from build123d import *

# Parameters (mm, degrees)
SKETCH1_W                                    = 20
SKETCH1_H                                    = 40
BOSS_EXTRUDE1_DEPTH                          = 3
CSK_FOR_M3_HEX_SOCKET_COUNTERSUNK_CA_2_COUNT = 2
CSK_FOR_M3_HEX_SOCKET_COUNTERSUNK_CA_2_PITCH = 10
CSK_FOR_M3_HEX_SOCKET_COUNTERSUNK_CA_3_COUNT = 2
CSK_FOR_M3_HEX_SOCKET_COUNTERSUNK_CA_3_PITCH = 18.027756377
CSK_FOR_M3_HEX_SOCKET_COUNTERSUNK_CA_4_COUNT = 2
CSK_FOR_M3_HEX_SOCKET_COUNTERSUNK_CA_4_PITCH = 15
M2_TAPPED_HOLE1_D                            = 1.6
BOSS_EXTRUDE2_DEPTH                          = 3
SKETCH7_W                                    = 30
SKETCH7_H                                    = 80.053183591
SKETCH7_R                                    = 2.65
BOSS_EXTRUDE3_DEPTH                          = 3
SKETCH8_R                                    = 2.65
BOSS_EXTRUDE4_DEPTH                          = 3
SKETCH9_R                                    = 2.6
CUT_EXTRUDE1_DEPTH                           = 4


with BuildPart() as part:
    # Sketch1 → Boss-Extrude1 (new body)
    with BuildSketch(Plane.XY):
        Rectangle(SKETCH1_W, SKETCH1_H)
    extrude(amount=BOSS_EXTRUDE1_DEPTH)

    # Sketch3 → CSK for M3 Hex Socket Countersunk Cap Screw1 (revolve, cut)
    with BuildSketch(Plane(origin=(-5, 0, 3), x_dir=(0, -1, 0), z_dir=(1, 0, 0))):
        Polygon((0, 0), (0, 3), (1.7, 3), (1.7, 1.66), (3.36, 0), align=None)
    csk_for_m3_hex_socket_countersunk_cap_sc = revolve(axis=Axis((-5, 0, 9.35), (0, 0, -1)), mode=Mode.SUBTRACT)

    # CSK for M3 Hex Socket Countersunk Ca 2: CSK for M3 Hex Socket Countersunk Cap Screw1 ×2
    with Locations(*[(i * CSK_FOR_M3_HEX_SOCKET_COUNTERSUNK_CA_2_PITCH, 0, 0) for i in range(1, CSK_FOR_M3_HEX_SOCKET_COUNTERSUNK_CA_2_COUNT)]):
        add(csk_for_m3_hex_socket_countersunk_cap_sc, mode=Mode.SUBTRACT)

    # CSK for M3 Hex Socket Countersunk Ca 3: CSK for M3 Hex Socket Countersunk Cap Screw1 ×2
    with Locations(*[Vector(0.554700196, -0.832050294, 0) * (i * CSK_FOR_M3_HEX_SOCKET_COUNTERSUNK_CA_3_PITCH) for i in range(1, CSK_FOR_M3_HEX_SOCKET_COUNTERSUNK_CA_3_COUNT)]):
        add(csk_for_m3_hex_socket_countersunk_cap_sc, mode=Mode.SUBTRACT)

    # CSK for M3 Hex Socket Countersunk Ca 4: CSK for M3 Hex Socket Countersunk Cap Screw1 ×2
    with Locations(*[(0, -i * CSK_FOR_M3_HEX_SOCKET_COUNTERSUNK_CA_4_PITCH, 0) for i in range(1, CSK_FOR_M3_HEX_SOCKET_COUNTERSUNK_CA_4_COUNT)]):
        add(csk_for_m3_hex_socket_countersunk_cap_sc, mode=Mode.SUBTRACT)

    # M2 Tapped Hole1 (through all)
    with Locations(Plane.XY.offset(3)):
        with Locations((0, 15), (0, 0), (0, -15)):
            Hole(M2_TAPPED_HOLE1_D / 2)

    # Sketch6 → Boss-Extrude2 (add)
    with BuildSketch(Plane.XY.offset(3)):
        Polygon((-10, 4), (-41, 4), (-41, 32), (10, 32), (10, 20), (-10, 20), align=None)
    extrude(amount=-BOSS_EXTRUDE2_DEPTH)

    # Sketch7 → Boss-Extrude3 (add)
    with BuildSketch(Plane.XY.offset(3)):
        with Locations((-10, 72.026591795)):
            Rectangle(SKETCH7_W, SKETCH7_H)
        with Locations((-19, 106.053183591)):
            Circle(SKETCH7_R, mode=Mode.SUBTRACT)
    extrude(amount=-BOSS_EXTRUDE3_DEPTH)

    # Sketch8 → Boss-Extrude4 (add)
    with BuildSketch(Plane.XY.offset(3)):
        Polygon((-25, 4), (-25, -35.5), (10, -35.5), (10, -20), (-10, -20), (-10, 4), align=None)
        with Locations((-19, -29.5)):
            Circle(SKETCH8_R, mode=Mode.SUBTRACT)
    extrude(amount=-BOSS_EXTRUDE4_DEPTH)

    # Sketch9 → Cut-Extrude1 (cut, through all)
    with BuildSketch(Plane.XY.offset(3)):
        with Locations((-18.5, 0)):
            Circle(SKETCH9_R)
        with Locations((-18.5, 36)):
            Circle(SKETCH9_R)
    extrude(amount=-CUT_EXTRUDE1_DEPTH, mode=Mode.SUBTRACT)


solid = part.part
Geometry check sheet. Reference: the model listing, model coordinates, mm. A direction names the side the tool comes from. Round coordinates to 2 decimals unless told otherwise and drop trailing zeros. Order: outer loops, then holes, each group sorted by start corner. A loop starts at its lowest first (then second) coordinate and runs counter-clockwise, first axis right, second up. Notation, with made-up numbers: (74, 26.5) -> (83, 26.5) arc R28 cw to (83, 57.5) -> close; hole circle Ø4 at (-31.5, 27). An arc over 180 degrees is marked (long way). Use one line per item in the form item = value.
1. Mould release check, pull along X, two halves, no side actions. Record for faces 4 (the face through (5, 71, 2)), 5 (the face through (-10, 39, 3)), 6 (the face through (6.5, -15.8, 0.7)): pulls with the +X half, pulls with the -X half, needs draft (parallel to the pull), parting line crosses it, or undercut.
Working result:
face_4 = pulls with the +X half
face_5 = needs draft
face_6 = undercut
2. Cross-section at B-B, the plane y = -29.5. Enter the section's corners in (x, z).
Working result:
outline = (-25, 0) -> (-21.65, 0) -> (-21.65, 3) -> (-25, 3) -> close; (-16.35, 0) -> (10, 0) -> (10, 3) -> (-16.35, 3) -> close
3. Set-up check for faces 1 (the face through (7, 32, 2)), 2 (the face through (-25, 71, 2)), 3 (the face through (-25, -15, 2)): record each of +Z, -Z, +X, -X, +Y, -Y from which the full face is reachable in a straight line by a thin tool's end or side.
Working result:
face_1 = +Z, -Z, +X, +Y
face_2 = +Z, -Z, -X, +Y
face_3 = +Z, -Z, -X, -Y
4. Cross-section at C-C, the plane z = 2.2. Count the separate pieces of the cut face and the enclosed holes in it, plus the area to 3 significant figures.
Working result:
separate_pieces = 1
enclosed_holes = 11
area = 5,040 mm^2
5. Scan lines: line 1 along Y through (x, z) = (0, 2.2); line 2 along Y through (x, z) = (-5, 1); line 3 along Y through (x, z) = (-19, 1.75). Record each from-to range of solid material in increasing order. Write a range as from..to.
Working result:
line_1 = -35.5..-15.8, -14.2..-0.8, 0.8..14.2, 15.8..112.05
line_2 = -35.5..-16.7, -13.3..-1.7, 1.7..112.05
line_3 = -35.5..-32.15, -26.85..-2.55, 2.55..33.45, 38.55..103.4, 108.7..112.05
6. Cross-section at D-D, the plane x = -19. Enter the section's corners in (y, z), plus the area to 3 significant figures.
Working result:
outline = (-35.5, 0) -> (-32.15, 0) -> (-32.15, 3) -> (-35.5, 3) -> close; (-26.85, 0) -> (-2.55, 0) -> (-2.55, 3) -> (-26.85, 3) -> close; (2.55, 0) -> (33.45, 0) -> (33.45, 3) -> (2.55, 3) -> close; (38.55, 0) -> (103.4, 0) -> (103.4, 3) -> (38.55, 3) -> close; (108.7, 0) -> (112.05, 0) -> (112.05, 3) -> (108.7, 3) -> close
area = 380 mm^2
7. Go/stop test with flat-tipped pins: pin 1 (4 mm diameter, centred on x = -5, y = 0, fed in from +Z); pin 2 (1.5 mm diameter, centred on x = 8, z = 1, fed in from +Y); pin 3 (3 mm diameter, centred on x = -18.5, y = 36, fed in from -Z); pin 4 (1.5 mm diameter, centred on y = 72.5, z = 2, fed in from -X). Record where each tip stops, or that it passes through.
Working result:
pin_1 = 1.64
pin_2 = 32
pin_3 = through
pin_4 = -25
8. Cross-section at A-A, the plane x = -5. Enter the section's corners in (y, z), plus the area to 3 significant figures.
Working result:
outline = (-35.5, 0) -> (-16.7, 0) -> (-16.7, 1.34) -> (-18.36, 3) -> (-35.5, 3) -> close; (-13.3, 0) -> (-1.7, 0) -> (-1.7, 1.34) -> (-3.36, 3) -> (-11.64, 3) -> (-13.3, 1.34) -> close; (1.7, 0) -> (112.05, 0) -> (112.05, 3) -> (3.36, 3) -> (1.7, 1.34) -> close
area = 417 mm^2
